Source: three-view drawing plus pictorial views. Frame: mm from the lowest corner of the part. A direction names the side the tool comes from. Coordinates: 2 decimals unless noted, no trailing zeros. Loops run counter-clockwise (first coordinate to the right, second up) from the corner with the lowest first, then second, coordinate; pieces in that order, holes last. Notation, with made-up numbers: (8, 26.5) - (57, 26.5) arc R9 cw to (57, 30.5) - close; hole circle Ø7 at (-6, 46). An arc over 180 degrees is marked (long way). Return JSON: item names as keys, results as strings.
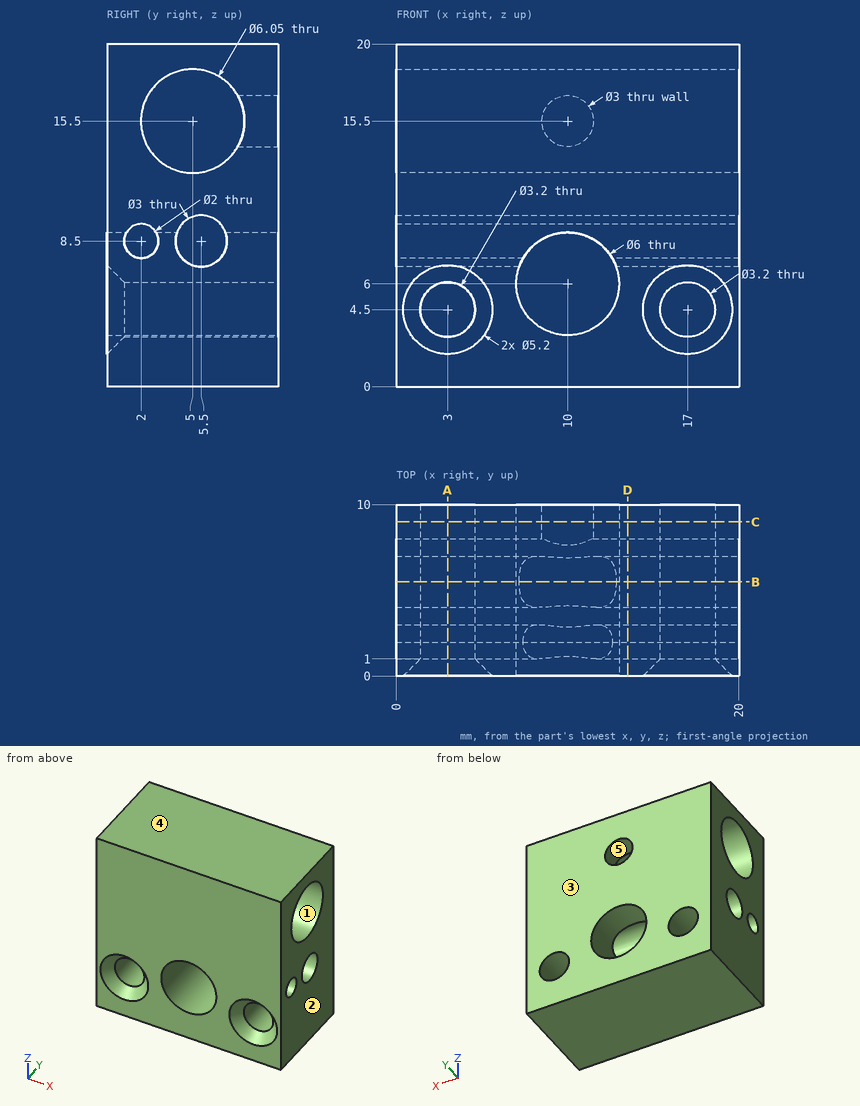
Item 1: Section query B-B, the plane y = 5.5. Return loops of the section in (x, z), and give its area (3 significant figures).
Worked out:
{"outline": "(0, 0) - (20, 0) - (20, 7) - (12.83, 7) arc R3 cw (long way) to (7.17, 7) - (0, 7) - close; (0, 10) - (20, 10) - (20, 12.52) - (0, 12.52) - close; (0, 18.48) - (20, 18.48) - (20, 20) - (0, 20) - close; hole circle Ø3.2 at (3, 4.5); hole circle Ø3.2 at (17, 4.5)", "area": "185 mm^2"}
Item 2: Section query C-C, the plane y = 9. Return loops of the section in (x, z).
Worked out:
{"outline": "(0, 0) - (20, 0) - (20, 20) - (0, 20) - close; hole circle Ø3.2 at (3, 4.5); hole circle Ø6 at (10, 6); hole circle Ø3 at (10, 15.5); hole circle Ø3.2 at (17, 4.5)"}
Item 3: Section query A-A, the plane x = 3. Return loops of the section in (y, z) (3 decimals).
Worked out:
{"outline": "(0, 0) - (10, 0) - (10, 2.9) - (1, 2.9) - (0, 1.9) - close; (0, 7.1) - (1, 6.1) - (10, 6.1) - (10, 20) - (0, 20) - close; hole circle Ø2 at (2, 8.5); hole circle Ø6.05 at (5, 15.5); hole circle Ø3 at (5.5, 8.5)"}
Item 4: Ray query, probe 1 along Z at (x, y) = (10, 8.6); probe 2 along Z at (x, y) = (6.75, 6); probe 3 along X at (y, z) = (1.5, 4). Return the intervals inside material, ascending. Write a range as from..to.
Worked out:
{"probe 1": "0..3, 9..14, 17..20", "probe 2": "0..7.09, 9.91..12.65, 18.35..20", "probe 3": "0..1.48, 4.52..7.76, 12.24..15.48, 18.52..20"}
Item 5: Mould query, pull axis Y, two halves, no side actions, for the marked faces 1, 2 and 3. Classes: +Y half, -Y half, draft (parallel to the pull), parting line (faces both ways), or undercut.
Worked out:
{"face 1": "undercut", "face 2": "draft", "face 3": "+Y half"}
Item 6: Reachability of the marked faces 4 and 5 from +Z, -Z, +X, -X, +Y, -Y: full face, straight path, thin tool, end or side. Return the list, or none.
Worked out:
{"face 4": "+Z, +X, -X, +Y, -Y", "face 5": "+Y"}
Item 7: Section query D-D, the plane x = 13.5. Return loops of the section in (y, z) (3 decimals).
Worked out:
{"outline": "(0, 0) - (10, 0) - (10, 20) - (0, 20) - close; hole circle Ø2 at (2, 8.5); hole circle Ø6.05 at (5, 15.5); hole circle Ø3 at (5.5, 8.5)"}
